Work out the finished part from the listing and answer in its coordinate system (mm). A direction names the side the tool comes from. Coordinates: 2 decimals unless noted, no trailing zeros. Order: outer loops, then holes, each group sorted by start corner. A loop starts at its lowest first (then second) coordinate and runs counter-clockwise, first axis right, second up. Notation, with made-up numbers: (54, -34.75) -> (108, -34.75) arc R16 cw to (108, -11.75) -> close; hole circle Ø2 at (69, -4.75). An arc over 180 degrees is marked (long way). Answer as CSV lines item,"result". Start each with the question number.
Item 1: Each of these flat-tipped pins is pushed along its axis until it touches: pin 1 Ø5 at (y, z) = (-1, 14) entering from -X; pin 2 Ø5 at (x, y) = (6.5, 5) entering from -Z; pin 3 Ø1.5 at (x, y) = (14, 0) entering from -Z; pin 4 Ø7.5 at (x, z) = (0, 0) entering from -Y. Where does it stop, or does it pass through?
Item 2: Section C-C (x = -10.5) is taken. Write down the section's boundary in (y, z), then the cut area to 3 significant figures.
Item 3: For a pull along X with two mould halves and no side action, classify faces 4 (the face through (22, 5, 2)), 5 (the face through (13.887, -2.465, -10.648)), 6 (the face through (-10.382, 8.521, -19.961)) as pulls with the +X half, pulls with the -X half, needs draft (parallel to the pull), parting line crosses it, or undercut.
Item 4: Which of the six approach directions +Z, -Z, +X, -X, +Y, -Y give full straight-line access (tool end or side, diameter ignored) to faces 1 (the face through (22, 7, 2)), 2 (the face through (13.887, 7.465, 10.648)), 3 (the face through (0, 0, -8))?
Item 5: Section A-A (y = -1.25) is taken. Write down the section's boundary in (x, z), then the cut area to 3 significant figures.
Item 6: Straight lines are drawn through the part: L1, parallel to Z at x = 0, y = 8.2; L2, parallel to Z at x = 0, y = 6; L3, parallel to Z at x = -4.5, y = 6.25. For each, find the intervals that lie inside material, in ascending order.
Item 7: Section B-B (z = -16) is taken. Write down the section's boundary in (x, y).
Item 8: Section D-D (y = 2.25) is taken. Write down the section's boundary in (x, z), then the cut area to 3 significant figures.
Autodesk Inventor part; units mm, degrees
ref_plane "YZ Plane" through (0, 0, 0) normal (1, 0, 0) x (0, 1, 0)
ref_plane "XZ Plane" through (0, 0, 0) normal (0, 1, 0) x (-1, 0, 0)
ref_plane "XY Plane" through (0, 0, 0) normal (0, 0, 1) x (1, 0, 0)
sketch "Sketch1" plane through (0, 0, 0) normal (0, 1, 0) x (-1, 0, 0)
  circle A0 centre (0, 0) radius 22.5
  circle A1 centre (0, 0) radius 2.55
  circle A2 centre (0, 0) radius 17.5
  circle A3 centre (0, 0) radius 21.5
  circle A4 centre (0, 0) radius 3.55
  dimension "d0" = 45
  dimension "d1" = 5.1
  dimension "d2" = 35
  dimension "d9" = 43
  dimension "d16" = 7.1
extrude "Extrusion1" add sketch "Sketch1" along normal blind 5 contours A2 | A4
extrude "Extrusion2" add sketch "Sketch1" along normal blind 10 contours A0 | A3
extrude "Extrusion3" add sketch "Sketch1" against normal blind 5 contours A0 | A3
extrude "Extrusion4" cut sketch "Sketch1" against normal blind 2 contours A0
sketch "Sketch2" plane through (0, 5, 0) normal (0, 1, 0) x (1, 0, 0)
  circle A0 centre (0, 0) radius 22.5
  circle A1 centre (0, 0) radius 21.5
  dimension "d12" = 45
  dimension "d13" = 43
extrude "Extrusion5" cut sketch "Sketch2" along normal blind 2
extrude "Extrusion6" add sketch "Sketch1" against normal blind 5 contours A4
extrude "Extrusion7" add sketch "Sketch1" along normal blind 10 contours A4
sketch "Sketch3" plane through (0, 10, 0) normal (0, 1, 0) x (1, 0, 0)
  circle A0 centre (0, 0) radius 4.05
  circle A1 centre (0, 0) radius 6
  dimension "d21" = 8.1
  dimension "d22" = 12
extrude "Extrusion8" add sketch "Sketch3" against normal blind 15
extrude "Extrusion9" cut sketch "Sketch3" against normal through all contours A0
properties part number "roller"
Checked values:
1,pin 1,"stops at x = -19.21"
1,pin 2,"stops at z = -22.14"
1,pin 3,"stops at z = -18.18"
1,pin 4,"passes through"
2,outline,"(-5, -19.9) -> (-2, -19.9) -> (-2, -18.76) -> (0, -18.76) -> (0, -19.9) -> (5, -19.9) -> (5, -18.76) -> (7, -18.76) -> (7, -19.9) -> (10, -19.9) -> (10, -14) -> (5, -14) -> (5, 14) -> (10, 14) -> (10, 19.9) -> (7, 19.9) -> (7, 18.76) -> (5, 18.76) -> (5, 19.9) -> (0, 19.9) -> (0, 18.76) -> (-2, 18.76) -> (-2, 19.9) -> (-5, 19.9) -> (-5, 14) -> (0, 14) -> (0, -14) -> (-5, -14) -> close"
2,area,"308 mm^2"
3,face 4,"needs draft"
3,face 5,"undercut"
3,face 6,"parting line crosses it"
4,face 1,"none"
4,face 2,"+Y"
4,face 3,"-Y"
5,outline,"circle Ø43 at (0, 0); circle Ø12 at (0, 0); hole circle Ø35 at (0, 0); hole circle Ø8.1 at (0, 0)"
5,area,"552 mm^2"
6,L1,"z = -22.5 to -17.5, -6 to -4.05, 4.05 to 6, 17.5 to 22.5"
6,L2,"z = -21.5 to -17.5, -6 to -4.05, 4.05 to 6, 17.5 to 21.5"
6,L3,"z = -21.02 to -16.91, -3.97 to 3.97, 16.91 to 21.02"
7,outline,"(-15.82, -5) -> (-7.09, -5) -> (-7.09, 0) -> (7.09, 0) -> (7.09, -5) -> (15.82, -5) -> (15.82, -2) -> (14.36, -2) -> (14.36, 0) -> (15.82, 0) -> (15.82, 5) -> (14.36, 5) -> (14.36, 7) -> (15.82, 7) -> (15.82, 10) -> (7.09, 10) -> (7.09, 5) -> (-7.09, 5) -> (-7.09, 10) -> (-15.82, 10) -> (-15.82, 7) -> (-14.36, 7) -> (-14.36, 5) -> (-15.82, 5) -> (-15.82, 0) -> (-14.36, 0) -> (-14.36, -2) -> (-15.82, -2) -> close"
8,outline,"circle Ø45 at (0, 0); hole circle Ø8.1 at (0, 0)"
8,area,"1,540 mm^2"
